Model file for the job. Use its own axes, mm. Face numbers are marked on the shaded views. A direction names the side the tool comes from. Coordinates: 2 decimals unless noted, no trailing zeros. Order: outer loops, then holes, each group sorted by start corner. A loop starts at its lowest first (then second) coordinate and runs counter-clockwise, first axis right, second up. Notation, with made-up numbers: M 88,-26 L 113,-26 A20 cw 113,8 Z; hole C -39.75,32 d3. An arc over 180 degrees is marked long. Return JSON: item names as keys, results as strings.
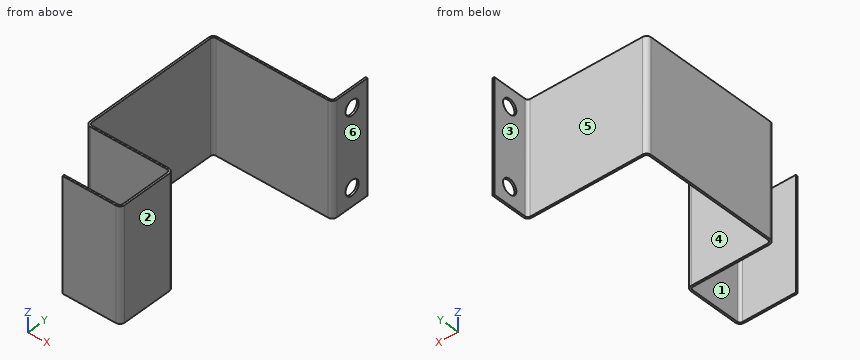
```python
from build123d import *

# Parameters (mm, degrees)
SKETCH1_W                    = 15
SKETCH1_H                    = 30.181487224
BASE_FLANGE2_DEPTH           = 0.5
EDGE_FLANGE1_STRIP_W         = 3.4732
EDGE_FLANGE1_STRIP_H         = 0.5
EDGE_FLANGE1_STRIP_CUT_DEPTH = 30.181487223
EDGE_FLANGE1_DEPTH           = 30.181487223
EDGE_FLANGE2_STRIP_W         = 3.4732
EDGE_FLANGE2_STRIP_H         = 0.5
EDGE_FLANGE2_STRIP_CUT_DEPTH = 30.181487223
EDGE_FLANGE2_DEPTH           = 30.181487223
EDGE_FLANGE6_STRIP_W         = 3.4732
EDGE_FLANGE6_STRIP_H         = 0.5
EDGE_FLANGE6_STRIP_CUT_DEPTH = 30.181487223
EDGE_FLANGE6_DEPTH           = 30.181487223
EDGE_FLANGE7_STRIP_W         = 3.4732
EDGE_FLANGE7_STRIP_H         = 0.5
EDGE_FLANGE7_STRIP_CUT_DEPTH = 30.181487223
EDGE_FLANGE7_DEPTH           = 30.181487223
EDGE_FLANGE8_STRIP_W         = 3.4732
EDGE_FLANGE8_STRIP_H         = 0.5
EDGE_FLANGE8_STRIP_CUT_DEPTH = 30.181487223
EDGE_FLANGE8_DEPTH           = 30.181487223
SKETCH58_R                   = 2
CUT_EXTRUDE1_DEPTH           = 74.128178856


# Sheet-metal steps are written as plain solids
with BuildPart() as part:
    # Sketch1 → Base-Flange2 (new body)
    with BuildSketch(Plane(origin=(0, 0, 0), x_dir=(1, 0, 0), z_dir=(0, 1, 0))):
        Rectangle(SKETCH1_W, SKETCH1_H)
    extrude(amount=BASE_FLANGE2_DEPTH)

    # Edge-Flange1 strip (across the edge) → Edge-Flange1 strip cut (cut)
    with BuildSketch(Plane(origin=(7.5, 0.5, 15.090743612), x_dir=(-1, 0, 0), z_dir=(0, 0, -1))):
        with Locations((-1, -0.25)):
            Rectangle(EDGE_FLANGE1_STRIP_W, EDGE_FLANGE1_STRIP_H)
    extrude(amount=EDGE_FLANGE1_STRIP_CUT_DEPTH, mode=Mode.SUBTRACT)

    # Edge-Flange1 section (across the edge) → Edge-Flange1 (add)
    with BuildSketch(Plane(origin=(7.5, 0.5, 15.090743612), x_dir=(-1, 0, 0), z_dir=(0, 0, -1))):
        with BuildLine():
            Line((-0.5, 0.7366), (-0.5, 15))
            Line((-0.5, 15), (0, 15))
            Line((0, 15), (0, 0.7366))
            ThreePointArc((0, 0.7366), (0.215745145, 0.215745145), (0.7366, 0))
            Line((0.7366, 0), (0.7366, -0.5))
            ThreePointArc((0.7366, -0.5), (-0.137808246, -0.137808246), (-0.5, 0.7366))
        make_face()
    extrude(amount=EDGE_FLANGE1_DEPTH)

    # Edge-Flange2 strip (across the edge) → Edge-Flange2 strip cut (cut)
    with BuildSketch(Plane(origin=(7.5, 15.5, 15.090743612), x_dir=(0, -1, 0), z_dir=(0, 0, -1))):
        with Locations((-1, -0.25)):
            Rectangle(EDGE_FLANGE2_STRIP_W, EDGE_FLANGE2_STRIP_H)
    extrude(amount=EDGE_FLANGE2_STRIP_CUT_DEPTH, mode=Mode.SUBTRACT)

    # Edge-Flange2 section (across the edge) → Edge-Flange2 (add)
    with BuildSketch(Plane(origin=(7.5, 15.5, 15.090743612), x_dir=(0, -1, 0), z_dir=(0, 0, -1))):
        with BuildLine():
            Line((-0.5, 0.7366), (-0.5, 22))
            Line((-0.5, 22), (0, 22))
            Line((0, 22), (0, 0.7366))
            ThreePointArc((0, 0.7366), (0.215745145, 0.215745145), (0.7366, 0))
            Line((0.7366, 0), (0.7366, -0.5))
            ThreePointArc((0.7366, -0.5), (-0.137808246, -0.137808246), (-0.5, 0.7366))
        make_face()
    extrude(amount=EDGE_FLANGE2_DEPTH)

    # Edge-Flange6 strip (across the edge) → Edge-Flange6 strip cut (cut)
    with BuildSketch(Plane(origin=(-14.5, 16, -15.090743612), x_dir=(1, 0, 0), z_dir=(0, 0, 1))):
        with Locations((-1, -0.25)):
            Rectangle(EDGE_FLANGE6_STRIP_W, EDGE_FLANGE6_STRIP_H)
    extrude(amount=EDGE_FLANGE6_STRIP_CUT_DEPTH, mode=Mode.SUBTRACT)

    # Edge-Flange6 section (across the edge) → Edge-Flange6 (add)
    with BuildSketch(Plane(origin=(-14.5, 16, -15.090743612), x_dir=(1, 0, 0), z_dir=(0, 0, 1))):
        with BuildLine():
            Line((-0.5, 0.7366), (-0.5, 37.5))
            Line((-0.5, 37.5), (0, 37.5))
            Line((0, 37.5), (0, 0.7366))
            ThreePointArc((0, 0.7366), (0.215745145, 0.215745145), (0.7366, 0))
            Line((0.7366, 0), (0.7366, -0.5))
            ThreePointArc((0.7366, -0.5), (-0.137808246, -0.137808246), (-0.5, 0.7366))
        make_face()
    extrude(amount=EDGE_FLANGE6_DEPTH)

    # Edge-Flange7 strip (across the edge) → Edge-Flange7 strip cut (cut)
    with BuildSketch(Plane(origin=(-14.5, 53.5, -15.090743612), x_dir=(0, -1, 0), z_dir=(0, 0, 1))):
        with Locations((-1, -0.25)):
            Rectangle(EDGE_FLANGE7_STRIP_W, EDGE_FLANGE7_STRIP_H)
    extrude(amount=EDGE_FLANGE7_STRIP_CUT_DEPTH, mode=Mode.SUBTRACT)

    # Edge-Flange7 section (across the edge) → Edge-Flange7 (add)
    with BuildSketch(Plane(origin=(-14.5, 53.5, -15.090743612), x_dir=(0, -1, 0), z_dir=(0, 0, 1))):
        with BuildLine():
            Line((-0.5, 0.7366), (-0.5, 31.5))
            Line((-0.5, 31.5), (0, 31.5))
            Line((0, 31.5), (0, 0.7366))
            ThreePointArc((0, 0.7366), (0.215745145, 0.215745145), (0.7366, 0))
            Line((0.7366, 0), (0.7366, -0.5))
            ThreePointArc((0.7366, -0.5), (-0.137808246, -0.137808246), (-0.5, 0.7366))
        make_face()
    extrude(amount=EDGE_FLANGE7_DEPTH)

    # Edge-Flange8 strip (across the edge) → Edge-Flange8 strip cut (cut)
    with BuildSketch(Plane(origin=(17, 54, 15.090743612), x_dir=(-1, 0, 0), z_dir=(0, 0, -1))):
        with Locations((-1, -0.25)):
            Rectangle(EDGE_FLANGE8_STRIP_W, EDGE_FLANGE8_STRIP_H)
    extrude(amount=EDGE_FLANGE8_STRIP_CUT_DEPTH, mode=Mode.SUBTRACT)

    # Edge-Flange8 section (across the edge) → Edge-Flange8 (add)
    with BuildSketch(Plane(origin=(17, 54, 15.090743612), x_dir=(-1, 0, 0), z_dir=(0, 0, -1))):
        with BuildLine():
            Line((-0.5, 0.7366), (-0.5, 10))
            Line((-0.5, 10), (0, 10))
            Line((0, 10), (0, 0.7366))
            ThreePointArc((0, 0.7366), (0.215745145, 0.215745145), (0.7366, 0))
            Line((0.7366, 0), (0.7366, -0.5))
            ThreePointArc((0.7366, -0.5), (-0.137808246, -0.137808246), (-0.5, 0.7366))
        make_face()
    extrude(amount=EDGE_FLANGE8_DEPTH)

    # Sketch58 → Cut-Extrude1 (cut, through all)
    with BuildSketch(Plane.ZY.offset(-17)):
        with Locations(Location((10.276185244, 59.3683, 0), (0, 0, 270))):
            Circle(SKETCH58_R)
        with Locations(Location((-10.276185244, 59.3683, 0), (0, 0, 90))):
            Circle(SKETCH58_R)
    extrude(amount=-CUT_EXTRUDE1_DEPTH, mode=Mode.SUBTRACT)


solid = part.part
```
Item 1: Wall check: line 1 (Y direction, x = -3.5, z = -3); line 2 (Y direction, x = -12, z = -12); line 3 (X direction, y = 20.5, z = 9). Give the ranges that are in metal, low to high.
Check result:
{"line 1": "y = 0 to 0.5, 15.5 to 16, 53.5 to 54", "line 2": "y = 15.5 to 16, 53.5 to 54", "line 3": "x = -15 to -14.5"}
Item 2: Saw through at B-B (z = 0.5). Write the cut outline in (x, y).
Check result:
{"outline": "M -15,16.74 A1.24 ccw -13.76,15.5 L 6.76,15.5 A0.74 cw 7.5,14.76 L 7.5,1.24 A0.74 cw 6.76,0.5 L -7.5,0.5 L -7.5,0 L 6.76,0 A1.24 ccw 8,1.24 L 8,14.76 A1.24 ccw 6.76,16 L -13.76,16 A0.74 cw -14.5,16.74 L -14.5,52.76 A0.74 cw -13.76,53.5 L 16.26,53.5 A1.24 ccw 17.5,54.74 L 17.5,64 L 17,64 L 17,54.74 A0.74 cw 16.26,54 L -13.76,54 A1.24 ccw -15,52.76 Z"}
Item 3: Saw through at D-D (y = 58.5). Write the cut outline in (x, z).
Check result:
{"outline": "M 17,-15.09 L 17.5,-15.09 L 17.5,-12.08 L 17,-12.08 Z; M 17,-8.47 L 17.5,-8.47 L 17.5,8.47 L 17,8.47 Z; M 17,12.08 L 17.5,12.08 L 17.5,15.09 L 17,15.09 Z"}
Item 4: Pull direction Y, two halves, no side cores. Call the marked faces 4, 5 and 6: +Y half, -Y half, draft (parallel to the pull), parting line (faces both ways), or undercut.
Check result:
{"face 4": "undercut", "face 5": "+Y half", "face 6": "draft"}
Item 5: Drop flat-ended pins along their axis: pin 1 Ø15 at (y, z) = (40, 4.5) entering from +X; pin 2 Ø2 at (x, z) = (10, -10) entering from -Y; pin 3 Ø6 at (x, z) = (-6, 3) entering from +Y. Give the stop position or say it passes through.
Check result:
{"pin 1": "stops at x = -14.5", "pin 2": "stops at y = 53.5", "pin 3": "stops at y = 54"}
Item 6: Saw through at A-A (x = -12). Write the cut outline in (y, z), and give its area (3 significant figures).
Check result:
{"outline": "M 15.5,-15.09 L 16,-15.09 L 16,15.09 L 15.5,15.09 Z; M 53.5,-15.09 L 54,-15.09 L 54,15.09 L 53.5,15.09 Z", "area": "30.2 mm2"}
Item 7: Saw through at C-C (x = 3). Write the cut outline in (y, z).
Check result:
{"outline": "M 0,-15.09 L 0.5,-15.09 L 0.5,15.09 L 0,15.09 Z; M 15.5,-15.09 L 16,-15.09 L 16,15.09 L 15.5,15.09 Z; M 53.5,-15.09 L 54,-15.09 L 54,15.09 L 53.5,15.09 Z"}
Item 8: 3-axis set-ups, long thin cutter, end or side, ignore diameter. For the marked faces 1, 2 and 3: which of +Z, -Z, +X, -X, +Y, -Y reach the whole face in a straight line?
Check result:
{"face 1": "+Z, -Z, -X", "face 2": "+Z, -Z, +X, -Y", "face 3": "+Z, -Z, -X, +Y"}
